Could you check a few things on this drawing? It's one solid part, dimensions in mm from its lowest x, y, z. A direction names the side the tool comes from. Give positions to 0.01 mm unless a question says otherwise; leave off trailing zeros. Order: outer loops, then holes, each group sorted by start corner. A loop starts at its lowest first (then second) coordinate and runs counter-clockwise, first axis right, second up. Notation, with made-up numbers: M -22.75,50.25 L 36.25,50.25 A32 cw 36.25,87.25 Z; hole C 58.5,-11.75 d8. An arc over 180 degrees is marked long. Use CSV: the item, a comma, the result in double quotes. Start each with the question number.
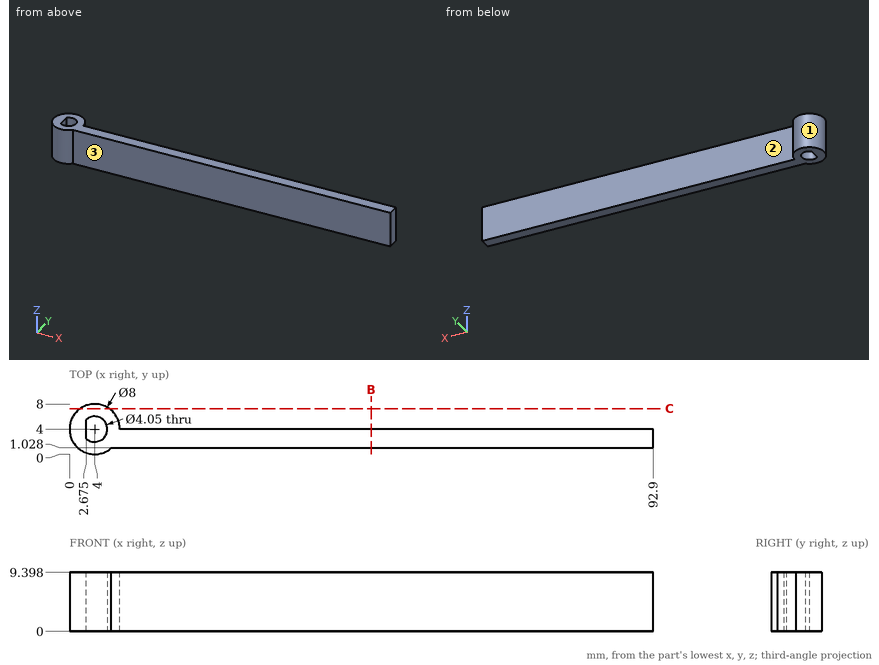
Q1. Imagine slicing it at B-B, the plane x = 48. Please give me the cut outline in (y, z).
Q2. I need wall thicknesses on line 1 (X direction, y = 4.25, z = 7.25) (1 decimal); line 2 (Y direction, x = 38, z = 4.5); line 3 (X direction, y = 0.5, z = 5) (1 decimal). Which ranges of each line are inside material? Lowest first, please. Write a range as [from, to].
Q3. For P1, Ø1.5, axis at x = 24, z = 3.5, coming from the +Y side, with a flat end and sliding along its axis, tell me the tip position at first contact or that it passes through.
Q4. For the marked faces 1, 2 and 3, which set-ups out of +Z, -Z, +X, -X, +Y, -Y let a thin tool reach every point of the face, with its end or its side?
Q5. Imagine slicing it at C-C, the plane y = 7.25. Please give me the cut outline in (x, z).
Reply:
1,outline,"M 1.03,0 L 4,0 L 4,9.4 L 1.03,9.4 Z"
2,line 1,"x = [0, 2.7], [6, 8]"
2,line 2,"y = [1.03, 4]"
2,line 3,"x = [2.1, 5.9]"
3,P1,"stops at y = 4"
4,face 1,"+Z, -Z"
4,face 2,"+Z, -Z, +X, +Y"
4,face 3,"+Z, -Z, +X, -Y"
5,outline,"M 1.67,0 L 6.33,0 L 6.33,9.4 L 1.67,9.4 Z"
